Build history of the part. All positions in model axes, mm. Give positions to 0.01 mm unless a question says otherwise; leave off trailing zeros. Loops run counter-clockwise (first coordinate to the right, second up) from the corner with the lowest first, then second, coordinate; pieces in that order, holes last. Notation, with made-up numbers: (43.25, 19.25) -> (99.25, 19.25) arc R26 cw to (99.25, 56.25) -> close; hole circle Ø9 at (-1, -30.75). An arc over 180 degrees is marked (long way). One line per question, with ' | ' between items. Start each with the question number.
(1) Flat gauge pins, fed straight in: pin 1 Ø7.5 at (x, y) = (69.5, 78) entering from +Z; pin 2 Ø3.5 at (x, y) = (44, 5) entering from +Z. Where does each tip first touch, or does it go through?
(2) Slice it at D-D, the plane z = 1.25. Give the number of separate pieces and of enclosed holes in the cut face, then the cut area to 3 significant figures.
(3) Slice it at B-B, the plane x = -20. Write the cut outline in (y, z).
(4) Drill centre lines: L1, parallel to Y at x = 44, z = 3.9; L2, parallel to Y at x = 5.5, z = 1; L3, parallel to X at y = 4.6, z = 1.8. Where is each one in solid material? Low to high. Write a range as from..to.
(5) Slice it at C-C, the plane y = 31. Write the cut outline in (x, z).
(6) Slice it at A-A, the plane x = 44. Write the cut outline in (y, z).
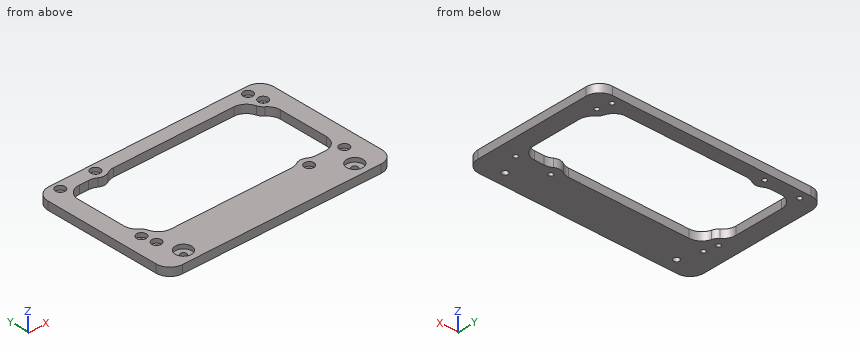
Autodesk Inventor part; units mm, degrees
ref_plane "YZ Plane" through (0, 0, 0) normal (1, 0, 0) x (0, 1, 0)
ref_plane "XZ Plane" through (0, 0, 0) normal (0, 1, 0) x (-1, 0, 0)
ref_plane "XY Plane" through (0, 0, 0) normal (0, 0, 1) x (1, 0, 0)
sketch "スケッチ1" plane through (0, 0, 0) normal (0, 0, 1) x (1, 0, 0)
  circle A0 centre (44, 4.4) radius 1.25 construction
  circle A1 centre (68, 78.4) radius 1.25 construction
  circle A2 centre (-70, 78.4) radius 1.25 construction
  circle A3 centre (-70, 14.4) radius 1.25 construction
  arc A4 (22.159, 26.4069) -> (22.159, 19.1931) centre (24.5, 22.8) ccw construction
  line L0 (22.159, 26.4069) -> (30.5, 31.8205) construction
  line L1 (30.5, 13.7795) -> (22.159, 19.1931) construction
  line L2 (58.5, 31.8205) -> (66.841, 26.4069) construction
  arc A5 (66.841, 19.1931) -> (66.841, 26.4069) centre (64.5, 22.8) ccw construction
  line L3 (58.5, 13.7795) -> (66.841, 19.1931) construction
  line L4 (35.3264, 11.8) -> (53.6736, 11.8) construction
  line L5 (73.8, 84.2) -> (-73.8, 84.2) construction
  line L6 (75, 83) -> (75, 9.6971) construction
  line L7 (-75, 5.3) -> (-75, 0) construction
  line L8 (75, 0) -> (75, 5.3) construction
  line L9 (-75, 84.2) -> (75, 84.2) construction
  line L10 (75, 84.2) -> (75, -1.2) construction
  line L11 (75, -1.2) -> (-75, -1.2) construction
  line L12 (-75, -1.2) -> (-75, 84.2) construction
  line L13 (-73, -1.2) -> (73, -1.2) construction
  line L14 (75, 84.2) -> (-75, -1.2) construction
  circle A6 centre (-70, 78.4) radius 1.7
  circle A7 centre (-70, 14.4) radius 1.7
  circle A8 centre (44, 4.4) radius 1.7
  circle A9 centre (68, 78.4) radius 1.7
  circle A10 centre (-70, 78.4) radius 7 construction
  circle A11 centre (-70, 14.4) radius 7 construction
  circle A12 centre (44, 4.4) radius 7 construction
  circle A13 centre (68, 78.4) radius 7 construction
  circle A14 centre (70, 4.6) radius 7 construction
  circle A15 centre (70, 4.6) radius 1.7
  circle A16 centre (70, 68.6) radius 7 construction
  circle A17 centre (70, 68.6) radius 1.7
  circle A18 centre (-44, 78.6) radius 7 construction
  circle A19 centre (-44, 78.6) radius 1.7
  circle A20 centre (-68, 4.6) radius 7 construction
  circle A21 centre (-68, 4.6) radius 1.7
  line L15 (-70, 74.2) -> (70, 74.2) construction
  line L16 (70, 74.2) -> (70, 8.8) construction
  line L17 (70, 8.8) -> (-70, 8.8) construction
  line L18 (-70, 8.8) -> (-70, 74.2) construction
  line L19 (90, 128.8) -> (-75, 128.8)
  line L20 (-75, 128.8) -> (-75, -1.2)
  line L21 (-75, -1.2) -> (90, -1.2)
  line L22 (90, -1.2) -> (90, 128.8)
  line L23 (-70, 71.4) -> (-70, 21.4)
  line L24 (-64.4, 74.2) -> (-49.4443, 74.2)
  line L25 (-38.5557, 74.2) -> (62.4, 74.2)
  line L26 (70, 61.6) -> (70, 11.6)
  line L27 (64.4, 8.8) -> (49.4443, 8.8)
  line L28 (38.5557, 8.8) -> (-62.4, 8.8)
  arc A22 (-64.201, 10.4794) -> (-70, 21.4) centre (-70, 14.4) ccw
  arc A23 (-62.4, 8.8) -> (-64.201, 10.4794) centre (-68, 4.6) ccw
  arc A24 (-70, 71.4) -> (-64.4, 74.2) centre (-70, 78.4) ccw
  arc A25 (-49.4443, 74.2) -> (-38.5557, 74.2) centre (-44, 78.6) ccw
  arc A26 (62.4, 74.2) -> (64.201, 72.5206) centre (68, 78.4) ccw
  arc A27 (64.201, 72.5206) -> (70, 61.6) centre (70, 68.6) ccw
  arc A28 (70, 11.6) -> (64.4, 8.8) centre (70, 4.6) ccw
  arc A29 (49.4443, 8.8) -> (38.5557, 8.8) centre (44, 4.4) ccw
  line L29 (-75, 84.2) -> (75, 84.2)
  line L30 (75, 84.2) -> (75, -1.2)
  point P0 (0, 0)
  point P1 (0, 41.5)
  point P2 (90, -1.2)
  point P3 (75, -1.2)
  dimension "d0" = 3.4
  dimension "d1" = 14
  dimension "d4" = 360
  dimension "d6" = 5
  dimension "d7" = 5
  dimension "d8" = 10
  dimension "d9" = 10
  dimension "d10" = 0
extrude "押し出し1" add sketch "スケッチ1" along normal blind 6 from surface at 0 contours L29 L30 L21 L20
ref_plane "作業平面3" through (1.1555, 128.8, 6) normal (0, 0, 1) x (1, 0, 0)
sketch "スケッチ6" plane through (1.1555, 128.8, 6) normal (0, 0, 1) x (1, 0, 0)
  circle A0 centre (-69.1555, -124.2) radius 1.7
  circle A1 centre (-71.1555, -114.4) radius 1.7
  circle A2 centre (-71.1555, -50.4) radius 1.7
  circle A3 centre (-45.1555, -50.2) radius 1.7
  circle A4 centre (66.8445, -50.4) radius 1.7
  circle A5 centre (68.8445, -60.2) radius 1.7
  circle A6 centre (68.8445, -124.2) radius 1.7
  circle A7 centre (42.8445, -124.4) radius 1.7
  circle A8 centre (-71.1555, -50.4) radius 3.5
  circle A9 centre (-71.1555, -114.4) radius 3.5
  circle A10 centre (-69.1555, -124.2) radius 3.5
  circle A11 centre (-45.1555, -50.2) radius 3.5
  circle A12 centre (66.8445, -50.4) radius 3.5
  circle A13 centre (68.8445, -60.2) radius 3.5
  circle A14 centre (68.8445, -124.2) radius 3.5
  circle A15 centre (42.8445, -124.4) radius 3.5
  point P0 (-1.1555, -128.8)
  dimension "d22" = 7
extrude "押し出し5" cut sketch "スケッチ6" along normal blind 10 and the other way blind 3 contours A0 | A1 | A2 | A3 | A4 | A5 | A6 | A7 | A8 | A9 | A10 | A11 | A12 | A13 | A14 | A15
sketch "スケッチ7" plane through (75, -1.2, 0) normal (0, 0, -1) x (-1, 0, 0)
  line L0 (150, 0) -> (150, 85.4)
  line L1 (0, 0) -> (150, 0)
  line L2 (0, 85.4) -> (0, 0)
  line L3 (150, 85.4) -> (158, 85.4)
  line L4 (158, 85.4) -> (158, -20)
  line L5 (158, -20) -> (-8, -20)
  line L6 (-8, -20) -> (-8, 85.4)
  line L7 (-8, 85.4) -> (0, 85.4)
  line L8 (158, -10) -> (-8, -10) construction
  circle A0 centre (12, -10) radius 2.25
  circle A1 centre (138, -10) radius 2.25
  point P0 (75, 1.2)
  dimension "d29" = 20
  dimension "d30" = 8
  dimension "d31" = 10
  dimension "d32" = 4.5
  dimension "d33" = 20
  dimension "d34" = 20
extrude "押し出し6" add sketch "スケッチ7" against normal up to surface (6 mm away)
fillet "フィレット4" radius 10 14 edges at (62.4, 74.2, 3) (64.201, 72.5206, 3) (70, 61.6, 3) (70, 11.6, 3) (64.4, 8.8, 3) (49.4443, 8.8, 3) (38.5557, 8.8, 3) (-62.4, 8.8, 3) (-64.201, 10.4794, 3) (-70, 21.4, 3) (-70, 71.4, 3) (-64.4, 74.2, 3) (-38.5557, 74.2, 3) (-49.4443, 74.2, 3)
fillet "フィレット5" radius 10 4 edges at (-83, 84.2, 3) (83, 84.2, 3) (83, -21.2, 3) (-83, -21.2, 3)
sketch "スケッチ8" plane through (-73, -21.2, 6) normal (0, 0, 1) x (1, 0, 0)
  circle A0 centre (10, 10) radius 2.25 construction
  circle A1 centre (136, 10) radius 2.25 construction
  circle A2 centre (10, 10) radius 6
  circle A3 centre (136, 10) radius 6
  point P0 (73, 21.2)
  dimension "d39" = 12
extrude "押し出し7" cut sketch "スケッチ8" against normal blind 3
equation "\"d7\" = d6"
equation "\"d9\" = d8"
equation "\"d31\" = 0.5 * d29"
equation "\"d34\" = d33"
properties part number "atx_power_holder"
Final values:
1) pin 1: z = 6 | pin 2: z = 3
2) separate pieces: 1 | enclosed holes: 11 | area: 8,440 mm2
3) outline: (-21.2, 0) -> (8.8, 0) -> (8.8, 6) -> (-21.2, 6) -> close; (74.2, 0) -> (84.2, 0) -> (84.2, 6) -> (74.2, 6) -> close
4) L1: -21.2..0.9, 7.9..11.4, 74.2..84.2 | L2: -21.2..8.8, 74.2..84.2 | L3: -83..-69.7, -66.3..42.31, 45.69..68.3, 71.7..83
5) outline: (-83, 0) -> (-70, 0) -> (-70, 6) -> (-83, 6) -> close; (70, 0) -> (83, 0) -> (83, 6) -> (70, 6) -> close
6) outline: (-21.2, 0) -> (2.7, 0) -> (2.7, 3) -> (0.9, 3) -> (0.9, 6) -> (-21.2, 6) -> close; (6.1, 0) -> (11.4, 0) -> (11.4, 6) -> (7.9, 6) -> (7.9, 3) -> (6.1, 3) -> close; (74.2, 0) -> (84.2, 0) -> (84.2, 6) -> (74.2, 6) -> close
